Part model, mm, in its own coordinate system. A direction names the side the tool comes from. Give positions to 0.01 mm unless a question says otherwise; leave off trailing zeros. Write each loop counter-clockwise with the first axis right and the second up, starting at its lowest first coordinate (ties: lowest second). Pieces come first, ordered by that corner, then holes. Notation, with made-up numbers: M 17,52 L 37,52 A5 ccw 37,61 Z; hole C 45,70.25 d2. An arc over 180 degrees is marked long. Answer as CSV lines item,"result". Start each with the question number.
1) Mould opens along X. For faces 4 (the flat face through (3.3, 13, -2.2)), 5 (the flat face through (0, 10, 0)), 6 (the flat face through (2.5, -1, 0)) say: pulls with the +X half, pulls with the -X half, needs draft (parallel to the pull), parting line crosses it, or undercut.
2) Slice it at D-D, the plane x = -0.75. Give the cut face in (y, z).
3) Pin check, flat tips, straight feed: pin 1 Ø4 at (x, y) = (-1, -4) entering from +Z; pin 2 Ø1.5 at (y, z) = (-2.5, 1) entering from -X; pin 3 Ø4 at (y, z) = (-2.5, -2) entering from +X; pin 4 Ø6 at (x, z) = (1, 2) entering from -Y. Stop position of each tip, or through.
4) Slice it at B-B, the plane x = -1.75. Give the cut face in (y, z), plus the area to 3 significant figures.
5) Wall check: line 1 along Y through (x, z) = (0, 2.1); line 2 along Z through (x, y) = (-0.75, -2.5); line 3 along X through (y, z) = (12.05, 0). Give the ranges that are in metal, low to high. Write a range as from..to.
6) Slice it at A-A, the plane z = 0. Give the cut face in (x, y), plus the area to 3 significant figures.
7) Tool access for faces 1 (the flat face through (0, -4, -1)), 2 (the flat face through (-2.5, -1, 0)), 3 (the flat face through (0, -4, -2.5)): list every direction of +Z, -Z, +X, -X, +Y, -Y with a clear straight run to the whole face (end or side of a thin tool).
```python
from build123d import *

# Parameters (mm, degrees)
SKETCH1_R           = 5
BOSS_EXTRUDE1_DEPTH = 13
SKETCH2_R           = 3.5
CUT_EXTRUDE1_DEPTH  = 3
SKETCH3_W           = 5
SKETCH3_H           = 5
BOSS_EXTRUDE2_DEPTH = 8
SKETCH4_W           = 5
SKETCH4_H           = 2
CUT_EXTRUDE2_DEPTH  = 6
FILLET2_R           = 2.5
SKETCH5_R           = 0.5
CUT_EXTRUDE4_DEPTH  = 16.81929202


with BuildPart() as part:
    # Sketch1 → Boss-Extrude1 (new body)
    with BuildSketch(Plane(origin=(0, 0, 0), x_dir=(1, 0, 0), z_dir=(0, 1, 0))):
        with Locations(Location((0, 0, 0), (0, 0, 90))):
            Circle(SKETCH1_R)
    extrude(amount=BOSS_EXTRUDE1_DEPTH)

    # Sketch2 → Cut-Extrude1 (cut)
    with BuildSketch(Plane(origin=(0, 13, 0), x_dir=(1, 0, 0), z_dir=(0, 1, 0))):
        with Locations(Location((0, 0, 0), (0, 0, 270))):
            Circle(SKETCH2_R)
    extrude(amount=-CUT_EXTRUDE1_DEPTH, mode=Mode.SUBTRACT)

    # Sketch3 → Boss-Extrude2 (add)
    with BuildSketch(Plane(origin=(0, 0, 0), x_dir=(-1, 0, 0), z_dir=(0, -1, 0))):
        Rectangle(SKETCH3_W, SKETCH3_H)
    extrude(amount=BOSS_EXTRUDE2_DEPTH)

    # Sketch4 → Cut-Extrude2 (cut)
    with BuildSketch(Plane(origin=(0, -8, 0), x_dir=(-1, 0, 0), z_dir=(0, -1, 0))):
        Rectangle(SKETCH4_W, SKETCH4_H)
    extrude(amount=-CUT_EXTRUDE2_DEPTH, mode=Mode.SUBTRACT)

    # Fillet2
    fillet2_edges = [part.edges().sort_by_distance(p)[0] for p in [
        (-2.5, -8, 1.75),
        (2.5, -8, 1.75),
        (2.5, -8, -1.75),
        (-2.5, -8, -1.75),
    ]]
    fillet(fillet2_edges, radius=FILLET2_R - 0.0001)  # a hair under: the kernel refuses the full size

    # Sketch5 → Cut-Extrude4 (cut, through all)
    with BuildSketch(Plane(origin=(0, 0, -2.5), x_dir=(-1, 0, 0), z_dir=(0, 0, -1))):
        with Locations((0, -5.5)):
            Circle(SKETCH5_R)
    extrude(amount=-CUT_EXTRUDE4_DEPTH, mode=Mode.SUBTRACT)


solid = part.part
```
Found:
1,face 4,"needs draft"
1,face 5,"undercut"
1,face 6,"pulls with the +X half"
2,outline,"M -7.88,-2.5 L 0,-2.5 L 0,-4.94 L 13,-4.94 L 13,-3.42 L 10,-3.42 L 10,3.42 L 13,3.42 L 13,4.94 L 0,4.94 L 0,2.5 L -7.88,2.5 L -7.88,1 L -2,1 L -2,-1 L -7.88,-1 Z"
3,pin 1,"z = 2.5"
3,pin 2,"x = -2.5"
3,pin 3,"x = 2.5"
3,pin 4,"y = -8"
4,outline,"M -7.29,-2.5 L 0,-2.5 L 0,-4.68 L 13,-4.68 L 13,-3.03 L 10,-3.03 L 10,3.03 L 13,3.03 L 13,4.68 L 0,4.68 L 0,2.5 L -7.29,2.5 L -7.29,1 L -2,1 L -2,-1 L -7.29,-1 Z"
4,area,"129 mm²"
5,line 1,"-8..-6, -5..10"
5,line 2,"-2.5..-1, 1..2.5"
5,line 3,"-5..-3.5, 3.5..5"
6,outline,"M -5,0 L -2.5,0 L -2.5,-2 L 2.5,-2 L 2.5,0 L 5,0 L 5,13 L 3.5,13 L 3.5,10 L -3.5,10 L -3.5,13 L -5,13 Z"
6,area,"119 mm²"
7,face 1,"+X, -X, -Y"
7,face 2,"+Z, -Z, -X, -Y"
7,face 3,"-Z, +X, -X, -Y"
